```python
from build123d import *

# Parameters (mm, degrees)
EXTRUDE1_DEPTH  = 460
LPATTERN1_COUNT = 8
LPATTERN1_PITCH = 60


with BuildPart() as part:
    # Sketch1 → Extrude1 (new body)
    with BuildSketch(Plane(origin=(-20, 0, 0), x_dir=(1, 0, 0), z_dir=(0, 0, 1))):
        with BuildLine():
            Line((12.5, 0.69999271), (13.199992786, 0))
            Line((13.199992786, 0), (26.800007214, 0))
            Line((26.800007214, 0), (27.5, 0.69999271))
            Line((27.5, 0.69999271), (27.5, 4.2000246))
            Line((27.5, 4.2000246), (24.8000183, 6.9000063))
            Line((24.8000183, 6.9000063), (24.8000183, 8.8400054))
            Line((24.8000183, 8.8400054), (25.755946813, 9.794179118))
            ThreePointArc((25.755946813, 9.794179118), (26.198484624, 10.690600567), (27.09432569, 11.13431209))
            Line((27.09432569, 11.13431209), (27.5, 11.5399866))
            Line((27.5, 11.5399866), (27.5, 12.8500204))
            Line((27.5, 12.8500204), (27.09432569, 13.268442751))
            ThreePointArc((27.09432569, 13.268442751), (26.202460867, 13.706434947), (25.755946813, 14.594063938))
            Line((25.755946813, 14.594063938), (25.3500197, 15))
            Line((25.3500197, 15), (14.6499803, 15))
            Line((14.6499803, 15), (14.244053187, 14.594063938))
            ThreePointArc((14.244053187, 14.594063938), (13.797539133, 13.706434947), (12.90567431, 13.268442751))
            Line((12.90567431, 13.268442751), (12.5, 12.8500204))
            Line((12.5, 12.8500204), (12.5, 11.5399866))
            Line((12.5, 11.5399866), (12.90567431, 11.13431209))
            ThreePointArc((12.90567431, 11.13431209), (13.801515376, 10.690600567), (14.244053187, 9.794179118))
            Line((14.244053187, 9.794179118), (15.1999817, 8.8400054))
            Line((15.1999817, 8.8400054), (15.1999817, 6.9000063))
            Line((15.1999817, 6.9000063), (12.5, 4.2000246))
            Line((12.5, 4.2000246), (12.5, 0.69999271))
        make_face()
    extrude(amount=-EXTRUDE1_DEPTH)

    # Sketch2 → Cut-Revolve1 (revolve, cut)
    with BuildSketch(Plane(origin=(0, 0, 0), x_dir=(0, 0, -1), z_dir=(1, 0, 0))):
        Polygon((20, 15), (23.75, 15), (23.75, 9.7), (22.25, 9.7), (22.25, 0), (20, 0), align=None)
    cut_revolve1 = revolve(axis=Axis((0, 0, -20), (0, 1, 0)), mode=Mode.SUBTRACT)

    # LPattern1: Cut-Revolve1 ×8
    with Locations(*[(0, 0, -i * LPATTERN1_PITCH) for i in range(1, LPATTERN1_COUNT)]):
        add(cut_revolve1, mode=Mode.SUBTRACT)


solid = part.part
```
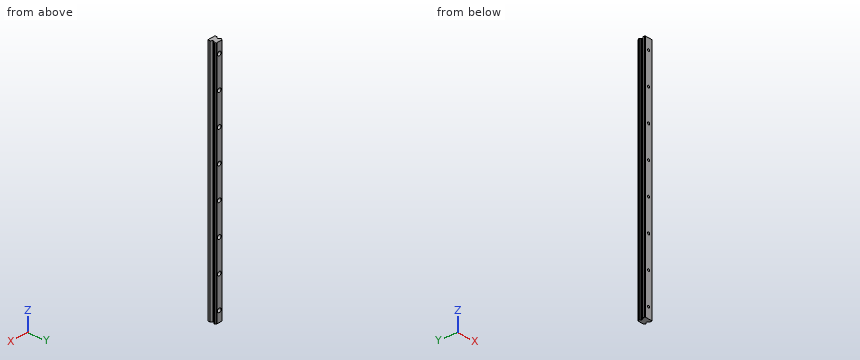
Can you work these out from the model? Positions are in its coordinate system, mm. Coordinates: 2 decimals unless noted, no trailing zeros. Loops run counter-clockwise (first coordinate to the right, second up) from the corner with the lowest first, then second, coordinate; pieces in that order, holes last. Notation, with made-up numbers: (63, -8) - (75, -8) arc R31 ccw to (75, 27) - close; hole circle Ø1 at (87, 74.5). An arc over 180 degrees is marked (long way). Answer as CSV lines item,"result". Start each with the question number.
1) Suppose I cut it at A-A (z = -54.5). Please give me the cut outline in (x, y).
2) I need wall thicknesses on line 1 (X direction, y = 11.95, z = -80); line 2 (X direction, y = 3.25, z = -380); line 3 (Y direction, x = 6.75, z = -294.5). Which ranges of each line are inside material? Lowest first, please. Write a range as from..to.
3) For pin 1 (6 mm diameter, centred on x = 0, z = -140, fed in from +Y); pin 2 (2 mm diameter, centred on y = 7.5, z = -77.5, fed in from +X); pin 3 (1.6 mm diameter, centred on y = 7.5, z = -261, fed in from -X), each with a flat end and sliding along its axis, tell me the tip position at first contact or that it passes through.
Check result:
1,outline,"(-7.5, 0.7) - (-6.8, 0) - (6.8, 0) - (7.5, 0.7) - (7.5, 4.2) - (4.8, 6.9) - (4.8, 8.84) - (5.76, 9.79) arc R1.56 cw to (7.09, 11.13) - (7.5, 11.54) - (7.5, 12.85) - (7.09, 13.27) arc R1.56 cw to (5.76, 14.59) - (5.35, 15) - (-5.35, 15) - (-5.76, 14.59) arc R1.56 cw to (-7.09, 13.27) - (-7.5, 12.85) - (-7.5, 11.54) - (-7.09, 11.13) arc R1.56 cw to (-5.76, 9.79) - (-4.8, 8.84) - (-4.8, 6.9) - (-7.5, 4.2) - close"
2,line 1,"x = -7.5..-3.75, 3.75..7.5"
2,line 2,"x = -7.5..-2.25, 2.25..7.5"
2,line 3,"y = 0..4.95, 11.05..13.36"
3,pin 1,"stops at y = 9.7"
3,pin 2,"stops at x = 5.2"
3,pin 3,"stops at x = -5"
